Here's how the part is built. I have some questions about the finished solid (model axes, mm). A direction names the side the tool comes from. Give positions to 0.01 mm unless a question says otherwise; leave off trailing zeros. Loops run counter-clockwise (first coordinate to the right, second up) from the corner with the lowest first, then second, coordinate; pieces in that order, holes last. Notation, with made-up numbers: M -36.75,41.5 L 18.25,41.5 A6 ccw 18.25,46.5 Z; hole C -20.5,49 d3. An arc over 180 degrees is marked long. Answer as CSV lines item,"result". Start each with the question number.
Item 1: I want a section at D-D on y = 17.5. List the corners of the cut face in (x, z) for me, plus the area to 3 significant figures.
Item 2: Will these pins go through, and if not, where does the flat tip stop? P1, Ø4, axis at x = 2.5, z = -14, coming from the -Y side; P2, Ø2.5, axis at y = 0, z = 0, coming from the +X side; P3, Ø4, axis at x = 6, z = -10, coming from the -Y side.
Item 3: If we mould it in two halves opening along Z, with no side actions, what happens to faces 1 (the flat face through (10.211, 0, -3)), 2 (the cylindrical face through (6.56, 0.53, 11.99)), 3 (the cylindrical face through (7, 0, 6))? For each: released by +Z, released by -Z, zero draft, split by the parting line, or undercut.
Item 4: For faces 4 (the cylindrical face through (5.77, -1.16, 1.51)), 5 (the cylindrical face through (7, -7, 9)), which set-ups out of +Z, -Z, +X, -X, +Y, -Y let a thin tool reach every point of the face, with its end or its side?
Item 5: I want a section at B-B on x = 7.25. List the corners of the cut face in (y, z) for me (3 decimals).
Item 6: I want a section at A-A on z = 0. List the corners of the cut face in (x, y) for me (3 decimals).
Item 7: If I drill on line 1 along Y through (x, z) = (8.5, 0) (3 decimals); line 2 along Z through (x, y) = (5.5, -1); line 3 along Z through (x, y) = (6.5, 2), over which ranges is the centre line in solid material (lowest first)? Write a range as from..to.
from build123d import *

# Parameters (mm, degrees)
SPROCKET_R                   = 45
ESTRUSIONE_ESTRUSIONE2_DEPTH = 3
SCHIZZO4_R                   = 10
ESTRUSIONE_ESTRUSIONE4_DEPTH = 12
SCHIZZO5_R                   = 20
SCHIZZO5_R_2                 = 19
ESTRUSIONE_ESTRUSIONE5_DEPTH = 12
SCHIZZO6_R                   = 3.175
TAGLIO_ESTRUSIONE1_DEPTH     = 16
SCALE1_SCALE                 = 0.6


with BuildPart() as part:
    # Sprocket → Estrusione-Estrusione2 (new body)
    with BuildSketch(Plane(origin=(0, 0, 0), x_dir=(0, 0, -1), z_dir=(1, 0, 0))):
        Circle(SPROCKET_R)
    extrude(amount=ESTRUSIONE_ESTRUSIONE2_DEPTH)

    # Schizzo4 → Estrusione-Estrusione4 (add)
    with BuildSketch(Plane(origin=(3, 0, 0), x_dir=(0, 0, -1), z_dir=(1, 0, 0))):
        Circle(SCHIZZO4_R)
    extrude(amount=ESTRUSIONE_ESTRUSIONE4_DEPTH)

    # Schizzo5 → Estrusione-Estrusione5 (add)
    with BuildSketch(Plane(origin=(3, 0, 0), x_dir=(0, 0, -1), z_dir=(1, 0, 0))):
        Circle(SCHIZZO5_R)
        Circle(SCHIZZO5_R_2, mode=Mode.SUBTRACT)
    extrude(amount=ESTRUSIONE_ESTRUSIONE5_DEPTH)

    # Schizzo6 → Taglio-Estrusione1 (cut, through all)
    with BuildSketch(Plane(origin=(15, 0, 0), x_dir=(0, 0, -1), z_dir=(1, 0, 0))):
        Circle(SCHIZZO6_R)
    extrude(amount=-TAGLIO_ESTRUSIONE1_DEPTH, mode=Mode.SUBTRACT)


with BuildPart() as part_1:
    # Scale1: scaled about (3.02832768, 0, 0)
    add(part.part.scale(SCALE1_SCALE).moved(Location((1.211331072, 0, 0))))


solid = part_1.part
Result:
1,outline,"M 1.21,-20.56 L 3.01,-20.56 L 3.01,20.56 L 1.21,20.56 Z"
1,area,"74.0 mm^2"
2,P1,"y = -24.19"
2,P2,"through"
2,P3,"y = -8.94"
3,face 1,"zero draft"
3,face 2,"split by the parting line"
3,face 3,"undercut"
4,face 4,"+X, -X"
4,face 5,"+X"
5,outline,"C 0,0 d24; C 0,0 d12; hole C 0,0 d22.8; hole C 0,0 d3.81"
6,outline,"M 1.211,-27 L 3.011,-27 L 3.011,-12 L 10.211,-12 L 10.211,-11.4 L 3.011,-11.4 L 3.011,-6 L 10.211,-6 L 10.211,-1.905 L 1.211,-1.905 Z; M 1.211,1.905 L 10.211,1.905 L 10.211,6 L 3.011,6 L 3.011,11.4 L 10.211,11.4 L 10.211,12 L 3.011,12 L 3.011,27 L 1.211,27 Z"
7,line 1,"-12..-11.4, -6..-1.905, 1.905..6, 11.4..12"
7,line 2,"-11.96..-11.36, -5.92..-1.62, 1.62..5.92, 11.36..11.96"
7,line 3,"-11.83..-11.22, -5.66..5.66, 11.22..11.83"
